```python
from build123d import *

# Parameters (mm, degrees)
SKETCH1_W           = 40
SKETCH1_H           = 40
BOSS_EXTRUDE1_DEPTH = 2
SKETCH2_R           = 1.5
CUT_EXTRUDE1_DEPTH  = 29.565713714
SKETCH3_W           = 4
SKETCH3_H           = 10
SKETCH3_W_2         = 10
SKETCH3_H_2         = 4
CUT_EXTRUDE2_DEPTH  = 29.565713714
SKETCH4_W           = 10
SKETCH4_H           = 4
BOSS_EXTRUDE2_DEPTH = 4
BOSS_EXTRUDE3_DEPTH = 4


with BuildPart() as part:
    # Sketch1 → Boss-Extrude1 (new, symmetric)
    with BuildSketch(Plane.XY):
        Rectangle(SKETCH1_W, SKETCH1_H)
    extrude(amount=BOSS_EXTRUDE1_DEPTH, both=True)

    # Sketch2 → Cut-Extrude1 (cut, through all)
    with BuildSketch(Plane.XY.offset(2)):
        with Locations((12, 14.35)):
            Circle(SKETCH2_R)
        with Locations((12, -3.15)):
            Circle(SKETCH2_R)
    extrude(amount=-CUT_EXTRUDE1_DEPTH, mode=Mode.SUBTRACT)

    # Sketch3 → Cut-Extrude2 (cut, through all)
    with BuildSketch(Plane.XY.offset(2)):
        with Locations((18, 10)):
            Rectangle(SKETCH3_W, SKETCH3_H)
        with Locations((-18, 10)):
            Rectangle(SKETCH3_W, SKETCH3_H)
        with Locations((-18, -10)):
            Rectangle(SKETCH3_W, SKETCH3_H)
        with Locations((18, -10)):
            Rectangle(SKETCH3_W, SKETCH3_H)
        with Locations((0, -8)):
            Rectangle(SKETCH3_W_2, SKETCH3_H_2)
    extrude(amount=-CUT_EXTRUDE2_DEPTH, mode=Mode.SUBTRACT)

    # Sketch4 → Boss-Extrude2 (add)
    with BuildSketch(Plane.XY.offset(2)):
        with Locations((-15, -22)):
            Rectangle(SKETCH4_W, SKETCH4_H)
        with Locations((15, -22)):
            Rectangle(SKETCH4_W, SKETCH4_H)
    extrude(amount=-BOSS_EXTRUDE2_DEPTH)

    # Sketch5 → Boss-Extrude3 (add)
    with BuildSketch(Plane.XY.offset(2)):
        Polygon((20, -20), (38, -20), (38, -24), (56, -24), (56, -20), (74, -20), (74, -24), (92, -24), (92, -20), (110, -20), (110, -10), (92, -10), (92, -6), (74, -6), (74, -10), (56, -10), (56, -6), (38, -6), (38, -10), (20, -10), align=None)
    extrude(amount=-BOSS_EXTRUDE3_DEPTH)


solid = part.part
```
Verification items for the finished model (mm, model axes). A direction names the side the tool comes from. Give positions to 0.01 mm unless a question says otherwise; leave off trailing zeros. Order: outer loops, then holes, each group sorted by start corner. A loop starts at its lowest first (then second) coordinate and runs counter-clockwise, first axis right, second up. Notation, with made-up numbers: (-20.5, 88.25) -> (-0.5, 88.25) arc R22 ccw to (-0.5, 104.25) -> close; hole circle Ø6 at (-35, 41). An arc over 180 degrees is marked (long way). Use a Markdown table: item, result.
1) Tool access check on faces 1 (the flat face through (-18, -5, 0)), 2 (the flat face through (29, -10, 0)), 3 (the flat face through (16, 10, 0)), 4 (the flat face through (0, -20, 0)), 5 (the flat face through (0, -10, 0)). Record the directions out of +Z, -Z, +X, -X, +Y, -Y that give a thin tool (end or side, any length) a straight path to the whole face; none if there is none.
Results:
| item | result |
|---|---|
| face 1 | +Z, -Z, -X |
| face 2 | +Z, -Z, +Y |
| face 3 | +Z, -Z, +X |
| face 4 | +Z, -Z, -Y |
| face 5 | +Z, -Z |
2) Depth check by flat-ended pin: pin 1 Ø1 at (x, z) = (27.5, 1) entering from -Y; pin 2 Ø1.2 at (y, z) = (-9, 0.5) entering from -X; pin 3 Ø1.2 at (x, z) = (82, 1) entering from +Y. Enter the tip coordinate at first touch or a pass-through.
Results:
| item | result |
|---|---|
| pin 1 | y = -20 |
| pin 2 | x = -16 |
| pin 3 | y = -6 |
3) Section check C-C, the plane z = 0.6. Give the number of separate pieces and of enclosed holes in the cut face, then the cut area to 3 significant figures.
Results:
| item | result |
|---|---|
| separate pieces | 1 |
| enclosed holes | 3 |
| area | 2,650 mm² |
4) Section check A-A, the plane x = 12. Record the boundary of the cut face in (y, z), then the cut area to 3 significant figures.
Results:
| item | result |
|---|---|
| outline | (-24, -2) -> (-4.65, -2) -> (-4.65, 2) -> (-24, 2) -> close; (-1.65, -2) -> (12.85, -2) -> (12.85, 2) -> (-1.65, 2) -> close; (15.85, -2) -> (20, -2) -> (20, 2) -> (15.85, 2) -> close |
| area | 152 mm² |
5) Section check B-B, the plane y = -3.15. Record the boundary of the cut face in (x, z), then the cut area to 3 significant figures.
Results:
| item | result |
|---|---|
| outline | (-20, -2) -> (10.5, -2) -> (10.5, 2) -> (-20, 2) -> close; (13.5, -2) -> (20, -2) -> (20, 2) -> (13.5, 2) -> close |
| area | 148 mm² |
6) Mould release check, pull along Y, two halves, no side actions. Record for faces 6 (the flat face through (10, -22, 0)), 7 (the flat face through (18, -5, 0)), 8 (the flat face through (15, -24, 0)), 9 (the flat face through (47, -6, 0)): pulls with the +Y half, pulls with the -Y half, needs draft (parallel to the pull), parting line crosses it, or undercut.
Results:
| item | result |
|---|---|
| face 6 | needs draft |
| face 7 | undercut |
| face 8 | pulls with the -Y half |
| face 9 | pulls with the +Y half |
7) Section check D-D, the plane y = 7. Record the boundary of the cut face in (x, z).
Results:
| item | result |
|---|---|
| outline | (-16, -2) -> (16, -2) -> (16, 2) -> (-16, 2) -> close |
8) Material ranges on probe 1 along Y at (x, z) = (12, 0); probe 2 along X at (y, z) = (-11.5, 1.15); probe 3 along X at (y, z) = (-8, 1.7), recorded low to high.
Results:
| item | result |
|---|---|
| probe 1 | -24 to -4.65, -1.65 to 12.85, 15.85 to 20 |
| probe 2 | -16 to 16, 20 to 110 |
| probe 3 | -16 to -5, 5 to 16, 38 to 56, 74 to 92 |
